from build123d import *
from build123d.topology import SkipClean

# Parameters (mm, degrees)
BOSS_EXTRUDE1_DEPTH = 1.4224
SKETCH2_R           = 3.81
BOSS_EXTRUDE2_DEPTH = 26.9875
SKETCH3_R           = 1.7526
CUT_EXTRUDE1_DEPTH  = 1.4224


with BuildPart() as part:
    # Sketch1 → Boss-Extrude1 (new body)
    with BuildSketch(Plane(origin=(0, 0, 0), x_dir=(1, 0, 0), z_dir=(0, 1, 0))):
        Polygon((0, 0), (26.9875, 0), (18.25625, 73.025), (8.73125, 73.025), align=None)
    extrude(amount=BOSS_EXTRUDE1_DEPTH)

    # Sketch2 → Boss-Extrude2 (add)
    with SkipClean():  # the faces are left unmerged after this step: merging them gives an invalid solid
        with BuildSketch(Plane(origin=(0, 0, 0), x_dir=(0, 0, -1), z_dir=(1, 0, 0))):
            with Locations((0, 3.81)):
                Circle(SKETCH2_R)
        extrude(amount=BOSS_EXTRUDE2_DEPTH)

    # Sketch3 → Cut-Extrude1 (cut)
    with SkipClean():  # the faces are left unmerged after this step: merging them gives an invalid solid
        with BuildSketch(Plane(origin=(0, 1.4224, 0), x_dir=(1, 0, 0), z_dir=(0, 1, 0))):
            with Locations(Location((13.49375, 63.5, 0), (0, 0, 270))):
                Circle(SKETCH3_R)
            with Locations(Location((7.9375, 12.7, 0), (0, 0, 270))):
                Circle(SKETCH3_R)
            with Locations(Location((19.05, 22.225, 0), (0, 0, 270))):
                Circle(SKETCH3_R)
        extrude(amount=-CUT_EXTRUDE1_DEPTH, mode=Mode.SUBTRACT)


solid = part.part
Part model, mm, in its own coordinate system. Give positions to 0.01 mm unless a question says otherwise; leave off trailing zeros. Write each loop counter-clockwise with the first axis right and the second up, starting at its lowest first coordinate (ties: lowest second). Pieces come first, ordered by that corner, then holes.
1) Pin check, flat tips, straight feed: pin 1 (4.5 mm diameter, centred on x = 19.05, z = -22.225, fed in from +Y); pin 2 (3 mm diameter, centred on y = 2.5, z = -10.5, fed in from -X); pin 3 (2 mm diameter, centred on x = 7.94, z = -12.7, fed in from +Y). Stop position of each tip, or through.
Resolved:
pin 1: stops at y = 1.42
pin 2: stops at x = 1.13
pin 3: passes through
2) Cut at B-B on x = 11. Write the cut outline in (y, z) (3 decimals).
Resolved:
outline: (0, -73.025) - (1.422, -73.025) - (1.422, -2.969) arc R3.81 ccw (long way) to (0, 0) - close
3) Cut at C-C on z = -22. Write the cut outline in (x, y).
Resolved:
outline: (2.63, 0) - (17.31, 0) - (17.31, 1.42) - (2.63, 1.42) - close; (20.79, 0) - (24.36, 0) - (24.36, 1.42) - (20.79, 1.42) - close
4) Probe L1, parallel to Z at x = 7.5, y = 3.5; L2, parallel to Z at x = 15, y = 1 (3 decimals); L3, parallel to Y at x = 6, z = -10. List the from-to ranges inside material, lowest first.
Resolved:
L1: z = -3.8 to 3.8
L2: z = -73.025 to -64.396, -62.604 to 2.573
L3: y = 0 to 1.42
5) Cut at A-A on z = -63.5. Write the cut outline in (x, y), then the cut area to 3 significant figures.
Resolved:
outline: (7.59, 0) - (11.74, 0) - (11.74, 1.42) - (7.59, 1.42) - close; (15.25, 0) - (19.4, 0) - (19.4, 1.42) - (15.25, 1.42) - close
area: 11.8 mm2
6) Two-plate mould, pull along Z, no slides. Class faces 1 (the face through (22.683, 0.701, -36.001)), 2 (the face through (6.87, 0.72, -14.09)), 3 (the face through (18.379, 0.721, -20.606)), 4 (the face through (13, 0, -29)): released by +Z, released by -Z, zero draft, split by the parting line, or undercut.
Resolved:
face 1: released by -Z
face 2: undercut
face 3: undercut
face 4: zero draft
7) Cut at D-D on y = 3. Write the cut outline in (x, z), then the cut area to 3 significant figures.
Resolved:
outline: (0, -3.72) - (26.99, -3.72) - (26.99, 3.72) - (0, 3.72) - close
area: 201 mm2
